The model under review builds one solid part; all positions refer to its coordinate system, in mm. A direction names the side the tool comes from. Coordinates: 2 decimals unless noted, no trailing zeros. Write each loop counter-clockwise with the first axis right and the second up, starting at its lowest first coordinate (ties: lowest second). Pieces come first, ordered by that corner, then holes.
```python
from build123d import *

# Parameters (mm, degrees)
SKETCH_W        = 150
SKETCH_H        = 130
SKETCH_R        = 3.75
SKETCH_R_2      = 1.75
SKETCH_W_2      = 110
SKETCH_H_2      = 68
PAD_DEPTH       = 3
SKETCH002_W     = 132
SKETCH002_H     = 77
POCKET001_DEPTH = 2.5
SKETCH007_W     = 5.5
SKETCH007_H     = 6
SKETCH007_R     = 2
PAD002_DEPTH    = 6
PAD003_DEPTH    = 10
SKETCH010_R     = 1.75
POCKET002_DEPTH = 6
SKETCH011_R     = 1.75
POCKET003_DEPTH = 7.5
SKETCH012_R     = 1.75
POCKET004_DEPTH = 7.5


with BuildPart() as part:
    # Sketch → Pad (new body)
    with BuildSketch(Plane.XY):
        with Locations((-75, -5)):
            Rectangle(SKETCH_W, SKETCH_H)
        with Locations((-27, -40.5)):
            Circle(SKETCH_R, mode=Mode.SUBTRACT)
        with Locations((-141, 45)):
            Circle(SKETCH_R_2, mode=Mode.SUBTRACT)
        with Locations((-141, -26)):
            Circle(SKETCH_R_2, mode=Mode.SUBTRACT)
        with Locations((-13.5, 45)):
            Circle(SKETCH_R_2, mode=Mode.SUBTRACT)
        with Locations((-13.5, -26)):
            Circle(SKETCH_R_2, mode=Mode.SUBTRACT)
        with Locations((-4, 56)):
            Circle(SKETCH_R_2, mode=Mode.SUBTRACT)
        with Locations((-4, -66)):
            Circle(SKETCH_R_2, mode=Mode.SUBTRACT)
        with Locations((-77, 11)):
            Rectangle(SKETCH_W_2, SKETCH_H_2, mode=Mode.SUBTRACT)
    extrude(amount=PAD_DEPTH)

    # Sketch002 → Pocket001 (cut)
    with BuildSketch(Plane.XY.offset(3.5)):
        with Locations((-77, 9.5)):
            Rectangle(SKETCH002_W, SKETCH002_H)
    extrude(amount=-POCKET001_DEPTH, mode=Mode.SUBTRACT)

    # Sketch007 → Pad002 (join)
    with BuildSketch(Plane.XY):
        with Locations((-141.25, 45)):
            Rectangle(SKETCH007_W, SKETCH007_H)
        with Locations((-141.5, 45)):
            Circle(SKETCH007_R, mode=Mode.SUBTRACT)
        with Locations((-13.75, 45)):
            Rectangle(SKETCH007_W, SKETCH007_H)
        with Locations((-13.5, 45)):
            Circle(SKETCH007_R, mode=Mode.SUBTRACT)
        with Locations((-13.75, -26)):
            Rectangle(SKETCH007_W, SKETCH007_H)
        with Locations((-13.5, -26)):
            Circle(SKETCH007_R, mode=Mode.SUBTRACT)
        with Locations((-141.25, -26)):
            Rectangle(SKETCH007_W, SKETCH007_H)
        with Locations((-141.5, -26)):
            Circle(SKETCH007_R, mode=Mode.SUBTRACT)
    extrude(amount=PAD002_DEPTH)

    # Sketch003 (on DatumPlane) → Pad003 (join)
    with BuildSketch(Plane.XY.offset(3)):
        Polygon((-20, 60), (-150, 60), (-150, -60), (-20, -60), (-20, -57), (-147, -57), (-147, 57), (-20, 57), align=None)
    extrude(amount=PAD003_DEPTH)

    # Sketch010 → Pocket002 (cut)
    with BuildSketch(Plane.XZ.offset(60)):
        with Locations((-125, 9.5)):
            Circle(SKETCH010_R)
        with Locations((-25, 9.5)):
            Circle(SKETCH010_R)
        with Locations((-75, 9.5)):
            Circle(SKETCH010_R)
    extrude(amount=-POCKET002_DEPTH, mode=Mode.SUBTRACT)

    # Sketch011 → Pocket003 (cut, symmetric)
    with BuildSketch(Plane.XZ.offset(-60)):
        with Locations((-75, 9.5)):
            Circle(SKETCH011_R)
        with Locations((-25, 9.5)):
            Circle(SKETCH011_R)
        with Locations((-125, 9.5)):
            Circle(SKETCH011_R)
    extrude(amount=POCKET003_DEPTH, both=True, mode=Mode.SUBTRACT)

    # Sketch012 (on DatumPlane) → Pocket004 (cut, symmetric)
    with BuildSketch(Plane.YZ.offset(-150)):
        with Locations((0, 9.5)):
            Circle(SKETCH012_R)
        with Locations((50, 9.5)):
            Circle(SKETCH012_R)
        with Locations((-50, 9.5)):
            Circle(SKETCH012_R)
    extrude(amount=POCKET004_DEPTH, both=True, mode=Mode.SUBTRACT)


solid = part.part
```
Item 1: For pin 1 (3 mm diameter, centred on x = -12.5, y = 46, fed in from +Z); pin 2 (2.5 mm diameter, centred on y = -26.5, z = 4.5, fed in from +X); pin 3 (2.5 mm diameter, centred on x = -14, z = 4.5, fed in from -Y), all flat-tipped, find the tip position at first contact; note any pin that passes through.
Solved:
pin 1: stops at z = 6
pin 2: stops at x = -11
pin 3: stops at y = -29
Item 2: Take a section at A-A, the plane x = -4. Write out the cut boundary in (y, z).
Solved:
outline: (-70, 0) - (-67.75, 0) - (-67.75, 3) - (-70, 3) - close; (-64.25, 0) - (54.25, 0) - (54.25, 3) - (-64.25, 3) - close; (57.75, 0) - (60, 0) - (60, 3) - (57.75, 3) - close
Item 3: Mouldability with a two-part tool opening along Z and no side actions: class faces 1 (the face through (-148, 0, 13)), 2 (the face through (-84, 57, 8)), 3 (the face through (-26.29, 58.52, 10.68)) as pulls with the +Z half, pulls with the -Z half, needs draft (parallel to the pull), parting line crosses it, or undercut.
Solved:
face 1: pulls with the +Z half
face 2: needs draft
face 3: undercut
Item 4: Machinability: for faces 4 (the face through (-14, 48, 4)), 5 (the face through (-83, -57, 8)), 6 (the face through (-139.592, -25.399, 3.625)), 7 (the face through (-16, 45, 6)), which of the approach directions +Z, -Z, +X, -X, +Y, -Y give a long, thin tool a straight path to every point of the face, cutting with its end or side? Answer none if there is none.
Solved:
face 4: +Z, +X, +Y
face 5: +Z, +X
face 6: +Z
face 7: +Z, +X, +Y, -Y
Item 5: Take a section at C-C, the plane y = 0. Write out the cut boundary in (x, z), plus the area to 3 significant figures.
Solved:
outline: (-150, 0) - (-132, 0) - (-132, 1) - (-143, 1) - (-143, 3) - (-147, 3) - (-147, 7.75) - (-150, 7.75) - close; (-150, 11.25) - (-147, 11.25) - (-147, 13) - (-150, 13) - close; (-22, 0) - (0, 0) - (0, 3) - (-11, 3) - (-11, 1) - (-22, 1) - close
area: 95.5 mm2
Item 6: To check wall thickness, follow line 1 along Y through (x, z) = (-13.5, 0.45); line 2 along X through (y, z) = (45, 3.25); line 3 along Y through (x, z) = (-13.5, 4.85). State the ranges of each line that lie inside material, in increasing order.
Solved:
line 1: y = -70 to -27.75, -24.25 to 43.25, 46.75 to 60
line 2: x = -150 to -147, -144 to -143.5, -139.5 to -138.5, -16.5 to -15.5, -11.5 to -11
line 3: y = -29 to -28, -24 to -23, 42 to 43, 47 to 48
Item 7: Take a section at B-B, the plane y = -40.5. Write out the cut boundary in (x, z).
Solved:
outline: (-150, 0) - (-30.75, 0) - (-30.75, 3) - (-147, 3) - (-147, 13) - (-150, 13) - close; (-23.25, 0) - (0, 0) - (0, 3) - (-23.25, 3) - close
Item 8: Take a section at D-D, the plane x = -70.5. Write out the cut boundary in (y, z), plus the area to 3 significant figures.
Solved:
outline: (-70, 0) - (-23, 0) - (-23, 1) - (-29, 1) - (-29, 3) - (-57, 3) - (-57, 13) - (-60, 13) - (-60, 3) - (-70, 3) - close; (45, 0) - (60, 0) - (60, 13) - (57, 13) - (57, 3) - (48, 3) - (48, 1) - (45, 1) - close
area: 228 mm2
